from build123d import *

# Parameters (mm, degrees)
F0_W     = 152.4
F0_H     = 76.073
F1_DEPTH = 50.8
F3_D     = 5.1054
F3_DEPTH = 16.51
F3_TIP   = 1.5338169022
F5_D     = 5.1054
F5_DEPTH = 16.51
F5_TIP   = 1.5338169022
F7_D     = 6.5278
F7_DEPTH = 16.9333333333
F7_TIP   = 1.9611489744


with BuildPart() as f1:
    # F0 (on Front) → F1 (new body)
    with BuildSketch(Plane.XZ):
        with Locations((-0.1111254096, 31.3906762446)):
            Rectangle(F0_W, F0_H)
    extrude(amount=F1_DEPTH)

    # F3
    with Locations(Plane(origin=(-76.3111254096, 0, 0), x_dir=(0, -1, 0), z_dir=(-1, 0, 0))):
        with Locations((25.4, 56.7271762446), (25.4, 5.9271762446)):
            Hole(F3_D / 2, depth=F3_DEPTH)
            with Locations((0, 0, -(F3_DEPTH + F3_TIP / 2))):  # 118° drill point
                Cone(0, F3_D / 2, F3_TIP, mode=Mode.SUBTRACT)

    # F5
    with Locations(Plane.YZ.offset(76.0888745904)):
        with Locations((-25.4, 56.7271762446), (-25.4, 6.0541762446)):
            Hole(F5_D / 2, depth=F5_DEPTH)
            with Locations((0, 0, -(F5_DEPTH + F5_TIP / 2))):  # 118° drill point
                Cone(0, F5_D / 2, F5_TIP, mode=Mode.SUBTRACT)

    # F7
    with Locations(Plane.XZ.offset(50.8)):
        with Locations((-38.2111254096, 31.3271762446), (37.9888745904, 31.3271762446)):
            Hole(F7_D / 2, depth=F7_DEPTH)
            with Locations((0, 0, -(F7_DEPTH + F7_TIP / 2))):  # 118° drill point
                Cone(0, F7_D / 2, F7_TIP, mode=Mode.SUBTRACT)


solid = f1.part
Could you check a few things on this model? Use its own coordinates, in mm. A direction names the side the tool comes from. Coordinates: 2 decimals unless noted, no trailing zeros.
Q1. Thinking about a two-plate mould opening in X: for faces 6 (the cylindrical face through (67.718, -24.847, 54.235)), 7 (the cylindrical face through (-34.95, -42.21, 31.47)), 8 (the conical face through (38.53, -32.246, 31.497)), 9 (the conical face through (58.311, -25.496, 56.294)), which applies, released by +X, released by -X, zero draft, split by the parting line, or undercut?
Q2. Which directions (+Z, -Z, +X, -X, +Y, -Y) give clear straight access to the entire face, cutting with the end or side of a thin tool? Please do faces 1 (the cylindrical face through (34.876, -42.215, 32.308)), 2 (the cylindrical face through (-67.94, -27.95, 6.04)), 3 (the flat face through (-1, 0, 32)), 4 (the flat face through (-76.311, -25, 31)), 5 (the cylindrical face through (67.72, -27.76, 5.08)).
Q3. Will these pins go through, and if not, where does the flat tip stop? pin 1 (1.5 mm diameter, centred on x = -60.5, z = 50.5, fed in from +Y); pin 2 (3 mm diameter, centred on y = -25.4, z = 5.93, fed in from +X); pin 3 (4.5 mm diameter, centred on y = -25.4, z = 56.73, fed in from -X); pin 4 (5 mm diameter, centred on x = -38.21, z = 31.33, fed in from -Y).
Q4. Please list where these lines run through material, in increasing order: L1, parallel to Z at x = 63, y = -25; L2, parallel to Z at x = -72.75, y = -25.4; L3, parallel to Y at x = 69.5, z = 57.5.
Answer:
1. face 6: zero draft
1. face 7: undercut
1. face 8: undercut
1. face 9: released by +X
2. face 1: -Y
2. face 2: -X
2. face 3: +Z, -Z, +X, -X, +Y
2. face 4: +Z, -Z, -X, +Y, -Y
2. face 5: +X
3. pin 1: stops at y = 0
3. pin 2: stops at x = 59.02
3. pin 3: stops at x = -59.62
3. pin 4: stops at y = -33.41
4. L1: z = -6.65 to 3.53, 8.58 to 54.21, 59.25 to 69.43
4. L2: z = -6.65 to 3.37, 8.48 to 54.17, 59.28 to 69.43
4. L3: y = -50.8 to -27.83, -22.97 to 0
